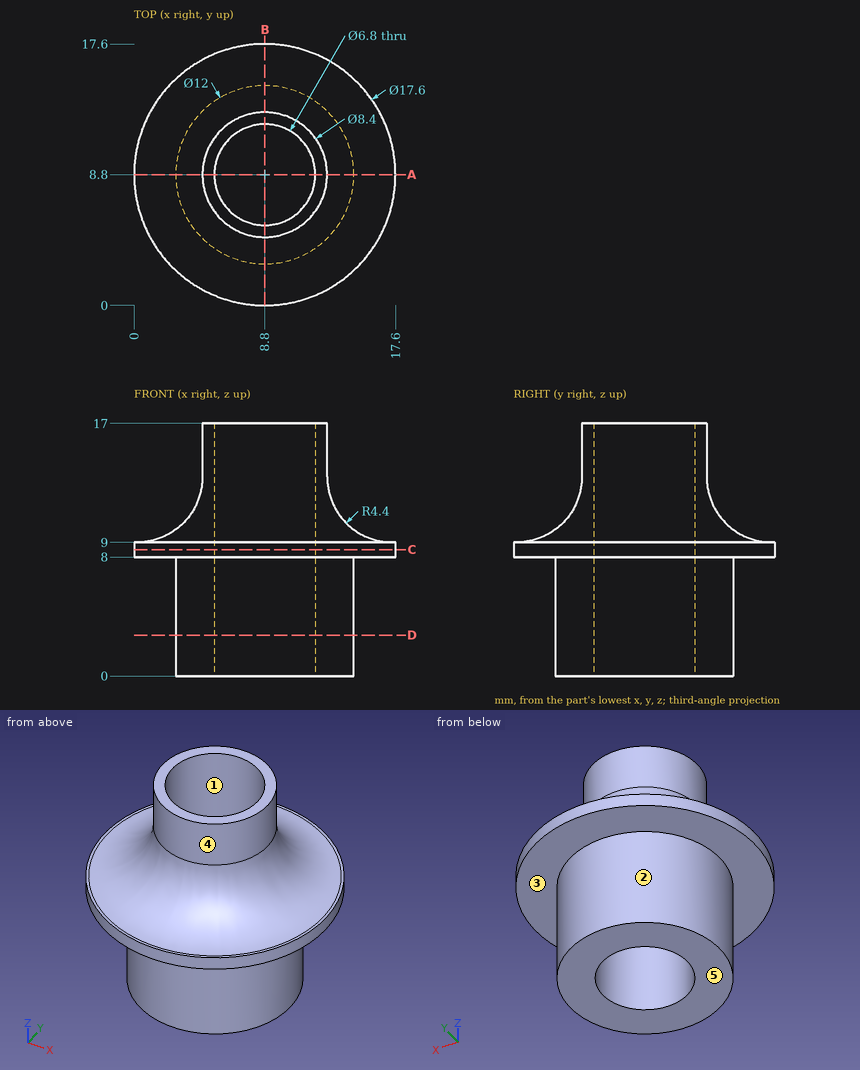
Job drawing, mm, ordinate dimensions from the low corner. One solid piece. A direction names the side the tool comes from. Coordinates: 2 decimals unless noted, no trailing zeros. Order: outer loops, then holes, each group sorted by start corner. A loop starts at its lowest first (then second) coordinate and runs counter-clockwise, first axis right, second up. Notation, with made-up numbers: M 62,85 L 101,85 A24 ccw 101,114 Z; hole C 14.25,2 d8. An arc over 180 degrees is marked long. Return JSON: item names as keys, results as strings.
1. Saw through at D-D (z = 2.75). Give the cut face in (x, y).
Ans:
{"outline": "C 8.8,8.8 d12; hole C 8.8,8.8 d6.8"}
2. Drill centre lines: probe 1 along Y at (x, z) = (8.8, 5.75); probe 2 along Y at (x, z) = (8.8, 9.5); probe 3 along X at (y, z) = (7.75, 12.75). Where is each one in solid material? Low to high.
Ans:
{"probe 1": "2.8 to 5.4, 12.2 to 14.8", "probe 2": "2.24 to 5.4, 12.2 to 15.36", "probe 3": "4.68 to 5.57, 12.03 to 12.92"}
3. Flat gauge pins, fed straight in: pin 1 (1.5 mm diameter, centred on x = 6.5, z = 3, fed in from -Y); pin 2 (5.5 mm diameter, centred on x = 8.8, y = 8.8, fed in from +Z) (1 decimal); pin 3 (5 mm diameter, centred on y = 4, z = 14, fed in from -X); pin 4 (4 mm diameter, centred on y = 10, z = 12.5, fed in from -X). Where does each tip first touch, or does it go through?
Ans:
{"pin 1": "y = 3", "pin 2": "through", "pin 3": "x = 5.29", "pin 4": "x = 3.6"}
4. Saw through at C-C (z = 8.5). Give the cut face in (x, y), and give its area (3 significant figures).
Ans:
{"outline": "C 8.8,8.8 d17.6; hole C 8.8,8.8 d6.8", "area": "207 mm^2"}
5. Saw through at A-A (y = 8.8). Give the cut face in (x, z).
Ans:
{"outline": "M 0,8 L 2.8,8 L 2.8,0 L 5.4,0 L 5.4,17 L 4.6,17 L 4.6,13.4 A4.4 cw 0.2,9 L 0,9 Z; M 12.2,0 L 14.8,0 L 14.8,8 L 17.6,8 L 17.6,9 L 17.4,9 A4.4 cw 13,13.4 L 13,17 L 12.2,17 Z"}
6. Pull direction X, two halves, no side cores. Call the marked faces 1, 2 and 3: +X half, -X half, draft (parallel to the pull), parting line (faces both ways), or undercut.
Ans:
{"face 1": "undercut", "face 2": "parting line", "face 3": "draft"}
7. Tool access for the marked faces 4 and 5: list every direction of +Z, -Z, +X, -X, +Y, -Y with a clear straight run to the whole face (end or side of a thin tool).
Ans:
{"face 4": "+Z", "face 5": "-Z, +X, -X, +Y, -Y"}
